For this review, take the finished solid that the model builds, in its own axes (mm). A direction names the side the tool comes from. Coordinates: 2 decimals unless noted, no trailing zeros. Order: outer loops, then holes, each group sorted by start corner. A loop starts at its lowest first (then second) coordinate and runs counter-clockwise, first axis right, second up. Notation, with made-up numbers: (87.25, -20) -> (124.25, -20) arc R13 ccw to (124.25, -8) -> close; hole circle Ø4 at (75.25, 86). An arc over 180 degrees is marked (long way). Write item = value, one per line. Start each with the question number.
1) Draft analysis for pull direction X (two halves, no side actions). For faces 5 (the face through (4, 4, 38)), 6 (the face through (-65, 59, 20)), 7 (the face through (71, 61, 5)), state which applies: +X half, -X half, draft (parallel to the pull), parting line (faces both ways), or undercut.
2) Wall thickness on probe 1 along X at (y, z) = (97, 19); probe 2 along X at (y, z) = (66.5, 24.5); probe 3 along Y at (x, z) = (67.5, 36.5): over which ranges is each line inside the solid? List them lowest first. Write a range as [from, to].
3) Machinability: for faces 1 (the face through (4, 116, 38)), 2 (the face through (4, 0, 18)), 3 (the face through (65, 56, 38)), 4 (the face through (-70, 59, 32)), which of the approach directions +Z, -Z, +X, -X, +Y, -Y give a long, thin tool a straight path to every point of the face, cutting with its end or side? Answer none if there is none.
4) Insertion check: pin 1 Ø1.2 at (x, z) = (63.5, 39) entering from -Y; pin 2 Ø4.5 at (x, z) = (-65.5, 37.5) entering from +Y; pin 3 Ø2.5 at (x, y) = (-71, 77) entering from -Z. Each pin has a flat end and moves straight along its axis. Give the tip position at first contact, or say it passes through.
5) Consider section A-A on z = 4. Give the boundary of the cut face in (x, y).
from build123d import *

# Parameters (mm, degrees)
F1_DEPTH    = 120
F2_SIZE2    = 2
F2_SIZE     = 5
F2_2_SIZE2  = 2
F2_2_SIZE   = 5
F3_T1_DEPTH = 162.2902937834
F3_T3_DEPTH = 166.2902937834
F4_T1_DEPTH = 125.1433659759
F4_T3_DEPTH = 137.1433659759
F4_T5_DEPTH = 122.2571417204
F10_DEPTH   = 120.001
F12_DEPTH   = 159.001


# Not quite as in the source:
# - a fillet or chamfer that OpenCascade refuses, or shapes differently, is made with other operations: its cross-section is extruded or revolved along the edge and cut away or added


with BuildPart() as f1:
    # F0 (on Front) → F1 (new body)
    with BuildSketch(Plane.XZ):
        Polygon((-75, 8), (-75, 0), (75, 0), (75, 10), (85, 10), (85, 30), (75, 30), (75, 40), (-75, 40), (-75, 32), (-65, 32), (-65, 8), align=None)
    extrude(amount=-F1_DEPTH)

    # F2
    f2_edges = [f1.edges().sort_by_distance(p)[0] for p in [
        (0, 0, 40),
    ]]
    f2_side = f1.faces().sort_by_distance((5.503356, 0, 20))[0]
    chamfer(f2_edges, length=F2_SIZE, length2=F2_SIZE2, reference=f2_side)

    # F2#2
    f2_2_edges = [f1.edges().sort_by_distance(p)[0] for p in [
        (0, 120, 40),
    ]]
    f2_2_side = f1.faces().sort_by_distance((5.503356, 120, 20))[0]
    chamfer(f2_2_edges, length=F2_2_SIZE, length2=F2_2_SIZE2, reference=f2_2_side)

    # F3: chamfer of 9 on 4 edges, made by hand

    # F3_s2 → F3_t1 (cut)
    with BuildSketch(Plane.XZ.offset(-141.1451468917)):
        Polygon((75, 31), (66, 40), (75, 40), align=None)
        Polygon((-66, 40), (-75, 31), (-75, 40), align=None)
    extrude(amount=F3_T1_DEPTH, mode=Mode.SUBTRACT)

    # F3_s4 → F3_t3 (cut)
    with BuildSketch(Plane.XZ.offset(-143.1451468917)):
        Polygon((-66, 0), (-75, 9), (-75, 0), align=None)
        Polygon((75, 9), (66, 0), (75, 0), align=None)
    extrude(amount=F3_T3_DEPTH, mode=Mode.SUBTRACT)

    # F4: chamfer of 1 on 6 edges, made by hand

    # F4_s2 → F4_t1 (cut)
    with BuildSketch(Plane.XZ.offset(-122.571682988)):
        Polygon((84, 30), (85, 29), (85, 30), align=None)
        Polygon((85, 11), (84, 10), (85, 10), align=None)
    extrude(amount=F4_T1_DEPTH, mode=Mode.SUBTRACT)

    # F4_s4 → F4_t3 (cut)
    with BuildSketch(Plane.YZ.offset(-68.571682988)):
        Polygon((0, 1), (1, 0), (0, 0), align=None)
        Polygon((120, 1), (119, 0), (120, 0), align=None)
    extrude(amount=F4_T3_DEPTH, mode=Mode.SUBTRACT)

    # F4_s6 → F4_t5 (cut)
    with BuildSketch(Plane.XZ.offset(-121.1285708602)):
        Polygon((-65.5857864376, 0), (-66.2928932188, 0.2928932188), (-66, 0), align=None)
        Polygon((66.2928932188, 0.2928932188), (65.5857864376, 0), (66, 0), align=None)
    extrude(amount=F4_T5_DEPTH, mode=Mode.SUBTRACT)

    # F6 (on offset) → F8 (revolve, cut)
    with BuildSketch(Plane.XY.offset(75)):
        with BuildLine():
            Line((-75, 60), (75, 60))
            add(Edge.make_bspline(
                [(75, 60), (75, 125), (0, 125), (-75, 125), (-75, 60)],
                knots=[0, 0, 0, 1.5707963268, 1.5707963268, 3.1415926536, 3.1415926536, 3.1415926536], degree=2, weights=[1, 0.7071067812, 1, 0.7071067812, 1]))
        make_face()
    revolve(axis=Axis((-0.8174791932, 60, 75), (1, 0, 0)), mode=Mode.SUBTRACT)

    # F9 (on face) → F10 (cut, through all)
    with BuildSketch(Plane.XZ):
        with BuildLine():
            Line((4, 36), (4, 40))
            Line((4, 40), (-4, 40))
            Line((-4, 40), (-4, 36))
            ThreePointArc((-4, 36), (0, 32), (4, 36))
        make_face()
    extrude(amount=-F10_DEPTH, mode=Mode.SUBTRACT)

    # F11 (on face) → F12 (cut, through all)
    with BuildSketch(Plane.YZ.offset(85)):
        with BuildLine():
            Line((64, 36.1), (64, 40))
            Line((64, 40), (56, 40))
            Line((56, 40), (56, 36.1))
            ThreePointArc((56, 36.1), (60, 32.1), (64, 36.1))
        make_face()
    extrude(amount=-F12_DEPTH, mode=Mode.SUBTRACT)


solid = f1.part
Answer sheet:
q1.face_5 = undercut
q1.face_6 = -X half
q1.face_7 = +X half
q2.probe_1 = [-65, 85]
q2.probe_2 = [-65, -46.62], [46.62, 85]
q2.probe_3 = [0.6, 56], [64, 119.4]
q3.face_1 = +Z, +Y, -Y
q3.face_2 = +Z, -Z, +X, -X, -Y
q3.face_3 = +Z, +X, -X
q3.face_4 = -X, +Y, -Y
q4.pin_1 = 1.36
q4.pin_2 = 119.9
q4.pin_3 = 3.75
q5.outline = (-70, 0) -> (70, 0) -> (70, 120) -> (-70, 120) -> close
